For this review, take the finished solid that the model builds, in its own axes (mm). A direction names the side the tool comes from. Give positions to 0.01 mm unless a question says otherwise; leave off trailing zeros. Order: outer loops, then holes, each group sorted by start corner. A loop starts at its lowest first (then second) coordinate and runs counter-clockwise, first axis right, second up. Notation, with made-up numbers: (-15.75, 48) - (-0.75, 48) arc R28 cw to (-0.75, 72) - close; hole circle Ø8 at (78, -26.5). An arc over 180 degrees is marked (long way). One line per item, written item: value.
```python
from build123d import *

# Parameters (mm, degrees)
SKETCH_2_W                       = 86
SKETCH_2_H                       = 1.5
SM_BASE_FLANGE_1_DEPTH           = 10
SM_EDGE_FLANGE_1_STRIP_W         = 7.4732
SM_EDGE_FLANGE_1_STRIP_H         = 1.5
SM_EDGE_FLANGE_1_STRIP_CUT_DEPTH = 86
SM_EDGE_FLANGE_1_DEPTH           = 86
SM_EDGE_FLANGE_2_STRIP_W         = 7.4732
SM_EDGE_FLANGE_2_STRIP_H         = 1.5
SM_EDGE_FLANGE_2_STRIP_CUT_DEPTH = 86
SM_EDGE_FLANGE_2_DEPTH           = 86
SKETCH_13_W                      = 50
SKETCH_13_H                      = 35
CUT_EXTRUDE_1_DEPTH              = 10
SKETCH_14_R                      = 2.072907101
CUT_EXTRUDE_2_DEPTH              = 104.111590037


# Sheet-metal steps are written as plain solids
with BuildPart() as part:
    # Sketch 2 → 基体-法兰1 (new body)
    with BuildSketch(Plane.XY):
        with Locations((43, -0.75)):
            Rectangle(SKETCH_2_W, SKETCH_2_H)
    extrude(amount=SM_BASE_FLANGE_1_DEPTH)

    # 边线-法兰1 strip (across the edge) → 边线-法兰1 strip cut (cut)
    with BuildSketch(Plane.ZY.offset(-86)):
        with Locations((-1.5, -0.75)):
            Rectangle(SM_EDGE_FLANGE_1_STRIP_W, SM_EDGE_FLANGE_1_STRIP_H)
    extrude(amount=SM_EDGE_FLANGE_1_STRIP_CUT_DEPTH, mode=Mode.SUBTRACT)

    # 边线-法兰1 section (across the edge) → 边线-法兰1 (add)
    with BuildSketch(Plane.ZY.offset(-86)):
        with BuildLine():
            Line((0, 0.7366), (0, 54.5))
            Line((0, 54.5), (1.5, 54.5))
            Line((1.5, 54.5), (1.5, 0.7366))
            ThreePointArc((1.5, 0.7366), (1.715745145, 0.215745145), (2.2366, 0))
            Line((2.2366, 0), (2.2366, -1.5))
            ThreePointArc((2.2366, -1.5), (0.655084973, -0.844915027), (0, 0.7366))
        make_face()
    extrude(amount=SM_EDGE_FLANGE_1_DEPTH)

    # 边线-法兰2 strip (across the edge) → 边线-法兰2 strip cut (cut)
    with BuildSketch(Plane(origin=(86, 54.5, 1.5), x_dir=(0, -1, 0), z_dir=(-1, 0, 0))):
        with Locations((-1.5, -0.75)):
            Rectangle(SM_EDGE_FLANGE_2_STRIP_W, SM_EDGE_FLANGE_2_STRIP_H)
    extrude(amount=SM_EDGE_FLANGE_2_STRIP_CUT_DEPTH, mode=Mode.SUBTRACT)

    # 边线-法兰2 section (across the edge) → 边线-法兰2 (add)
    with BuildSketch(Plane(origin=(86, 54.5, 1.5), x_dir=(0, -1, 0), z_dir=(-1, 0, 0))):
        with BuildLine():
            Line((0, 0.7366), (0, 8.5))
            Line((0, 8.5), (1.5, 8.5))
            Line((1.5, 8.5), (1.5, 0.7366))
            ThreePointArc((1.5, 0.7366), (1.715745145, 0.215745145), (2.2366, 0))
            Line((2.2366, 0), (2.2366, -1.5))
            ThreePointArc((2.2366, -1.5), (0.655084973, -0.844915027), (0, 0.7366))
        make_face()
    extrude(amount=SM_EDGE_FLANGE_2_DEPTH)

    # 草图13 → 切除-拉伸1 (cut)
    with BuildSketch(Plane(origin=(0, 0, 0), x_dir=(-1, 0, 0), z_dir=(0, 0, -1))):
        with Locations((-43, 26.5)):
            Rectangle(SKETCH_13_W, SKETCH_13_H)
    extrude(amount=-CUT_EXTRUDE_1_DEPTH, mode=Mode.SUBTRACT)

    # 草图14 → 切除-拉伸2 (cut, through all)
    with BuildSketch(Plane(origin=(0, 54.5, 0), x_dir=(1, 0, 0), z_dir=(0, 1, 0))):
        with Locations(Location((15.5, -5.5, 0), (0, 0, 270))):
            Circle(SKETCH_14_R)
        with Locations(Location((70.5, -5.5, 0), (0, 0, 270))):
            Circle(SKETCH_14_R)
    extrude(amount=-CUT_EXTRUDE_2_DEPTH, mode=Mode.SUBTRACT)


solid = part.part
```
(1) Wall thickness on line 1 (X direction, y = 54.1, z = 5.5); line 2 (Y direction, x = 14, z = 3.75); line 3 (X direction, y = 41, z = 0.5): over which ranges is each line inside the solid? List them lowest first. Write a range as from..to.
Answers below:
line 1: x = 0..13.43, 17.57..68.43, 72.57..86
line 2: y = -1.5..0, 53..54.5
line 3: x = 0..18, 68..86
(2) For P1, Ø4, axis at x = 12, y = 38, coming from the -Z side; P2, Ø1.2, axis at x = 52.5, z = 1, coming from the +Y side; P3, Ø2.5, axis at x = 15.5, z = 5.5, coming from the +Y side; P4, Ø1.2, axis at x = 38, z = 1, coming from the -Y side, all flat-tipped, find the tip position at first contact; note any pin that passes through.
Answers below:
P1: stops at z = 0
P2: stops at y = 54.41
P3: passes through
P4: stops at y = -1.41
(3) Take a section at B-B (y = 36). Write out the cut boundary in (x, z), then the cut area to 3 significant figures.
Answers below:
outline: (0, 0) - (18, 0) - (18, 1.5) - (0, 1.5) - close; (68, 0) - (86, 0) - (86, 1.5) - (68, 1.5) - close
area: 54.0 mm^2
(4) Machinability: for faces 1 (the face through (42, 0, 6)), 2 (the face through (44, 3, 0)), which of the approach directions +Z, -Z, +X, -X, +Y, -Y give a long, thin tool a straight path to every point of the face, cutting with its end or side? Answer none if there is none.
Answers below:
face 1: +Z, +X, -X
face 2: -Z, +X, -X, +Y, -Y
(5) Take a section at D-D (x = 46). Write out the cut boundary in (y, z).
Answers below:
outline: (-1.5, 2.24) arc R2.24 ccw to (0.74, 0) - (9, 0) - (9, 1.5) - (0.74, 1.5) arc R0.74 cw to (0, 2.24) - (0, 10) - (-1.5, 10) - close; (44, 0) - (52.26, 0) arc R2.24 ccw to (54.5, 2.24) - (54.5, 10) - (53, 10) - (53, 2.24) arc R0.74 cw to (52.26, 1.5) - (44, 1.5) - close
(6) Draft analysis for pull direction Z (two halves, no side actions). For faces 3 (the face through (43.6, -0.86, 0.67)), 4 (the face through (44, 53, 6)), 5 (the face through (13.476, 53.76, 5.051)), 6 (the face through (13.476, -0.739, 5.051)), state which applies: pulls with the +Z half, pulls with the -Z half, needs draft (parallel to the pull), parting line crosses it, or undercut.
Answers below:
face 3: pulls with the -Z half
face 4: needs draft
face 5: undercut
face 6: undercut
(7) Take a section at A-A (x = 70.5). Write out the cut boundary in (y, z).
Answers below:
outline: (-1.5, 2.24) arc R2.24 ccw to (0.74, 0) - (52.26, 0) arc R2.24 ccw to (54.5, 2.24) - (54.5, 3.43) - (53, 3.43) - (53, 2.24) arc R0.74 cw to (52.26, 1.5) - (0.74, 1.5) arc R0.74 cw to (0, 2.24) - (0, 3.43) - (-1.5, 3.43) - close; (-1.5, 7.57) - (0, 7.57) - (0, 10) - (-1.5, 10) - close; (53, 7.57) - (54.5, 7.57) - (54.5, 10) - (53, 10) - close
(8) Take a section at C-C (z = 5.5). Write out the cut boundary in (x, y), then the cut area to 3 significant figures.
Answers below:
outline: (0, -1.5) - (13.43, -1.5) - (13.43, 0) - (0, 0) - close; (0, 53) - (13.43, 53) - (13.43, 54.5) - (0, 54.5) - close; (17.57, -1.5) - (68.43, -1.5) - (68.43, 0) - (17.57, 0) - close; (17.57, 53) - (68.43, 53) - (68.43, 54.5) - (17.57, 54.5) - close; (72.57, -1.5) - (86, -1.5) - (86, 0) - (72.57, 0) - close; (72.57, 53) - (86, 53) - (86, 54.5) - (72.57, 54.5) - close
area: 233 mm^2
